Design review of the part built by this model. Coordinates are the model's own, in mm. A direction names the side the tool comes from. Coordinates: 2 decimals unless noted, no trailing zeros. Order: outer loops, then holes, each group sorted by start corner. A loop starts at its lowest first (then second) coordinate and runs counter-clockwise, first axis right, second up. Notation, with made-up numbers: (88.25, 33) - (121.25, 33) arc R12 ccw to (121.25, 52) - close; hole circle Ø4 at (22, -10.5). An arc over 180 degrees is marked (long way). Write item = value, one per line. Start each with the question number.
```python
from build123d import *

# Parameters (mm, degrees)
SKETCH_1_R               = 8.5
EXTRUDE_1_DEPTH          = 15
SKETCH_2_R               = 10
EXTRUDE_2_DEPTH          = 10
SKETCH_3_R               = 1
CUT_EXTRUDE_1_DEPTH      = 10
CUT_EXTRUDE_START        = -1.9
SKETCH_4_R               = 8.5
SKETCH_4_R_2             = 8.1
CUT_EXTRUDE_2_DEPTH      = 1.6
CHAMFER_1_SIZE           = 0.5
SKETCH_7_R               = 1
CUT_EXTRUDE_3_DEPTH      = 8
PATTERN_CIRCULAR_1_COUNT = 4
SKETCH_8_R               = 3.5
CUT_EXTRUDE_4_DEPTH      = 5.5
CHAMFER_2_SIZE           = 0.5
CUT_EXTRUDE_5_REACH      = 21.5
SKETCH_9_R               = 2.5


with BuildPart() as part:
    # Эскиз1 → Бобышка-Вытянуть1 (new body)
    with BuildSketch(Plane(origin=(0, 0, 0), x_dir=(1, 0, 0), z_dir=(0, 1, 0))):
        Circle(SKETCH_1_R)
    extrude(amount=EXTRUDE_1_DEPTH)

    # Эскиз2 → Бобышка-Вытянуть2 (add)
    with BuildSketch(Plane(origin=(0, 15, 0), x_dir=(1, 0, 0), z_dir=(0, 1, 0))):
        Circle(SKETCH_2_R)
    extrude(amount=EXTRUDE_2_DEPTH)

    # Эскиз3 → Вырез-Вытянуть1 (cut)
    with BuildSketch(Plane.XZ):
        with Locations((0, 6)):
            Circle(SKETCH_3_R)
        with Locations((6, 0)):
            Circle(SKETCH_3_R)
        with Locations((0, -6)):
            Circle(SKETCH_3_R)
        with Locations((-6, 0)):
            Circle(SKETCH_3_R)
    extrude(amount=-CUT_EXTRUDE_1_DEPTH, mode=Mode.SUBTRACT)

    # Эскиз4 → Вырез-Вытянуть2 (cut)
    with BuildSketch(Plane.XZ.offset(CUT_EXTRUDE_START)):
        Circle(SKETCH_4_R)
        Circle(SKETCH_4_R_2, mode=Mode.SUBTRACT)
    extrude(amount=-CUT_EXTRUDE_2_DEPTH, mode=Mode.SUBTRACT)

    # Фаска1
    chamfer_1_edges = [part.edges().sort_by_distance(p)[0] for p in [
        (-8.5, 0, 0),
        (-10, 25, 0),
    ]]
    chamfer(chamfer_1_edges, length=CHAMFER_1_SIZE)

    # Эскиз7 → Вырез-Вытянуть3 (cut)
    with BuildSketch(Plane(origin=(6.524591557, 0, 7.578238913), x_dir=(0.757823891, 0, -0.652459156), z_dir=(0.652459156, 0, 0.757823891))):
        with Locations((0, 22)):
            Circle(SKETCH_7_R)
    cut_extrude_3 = extrude(amount=-CUT_EXTRUDE_3_DEPTH, mode=Mode.SUBTRACT)

    # Круговой массив1: Вырез-Вытянуть3 ×4 about axis
    pattern_circular_1_axis = Axis((0, 0, 0), (0, 1, 0))
    for i in range(1, PATTERN_CIRCULAR_1_COUNT):
        add(cut_extrude_3.rotate(pattern_circular_1_axis, i * 360 / PATTERN_CIRCULAR_1_COUNT), mode=Mode.SUBTRACT)

    # Эскиз8 → Вырез-Вытянуть4 (cut)
    with BuildSketch(Plane.XZ):
        Circle(SKETCH_8_R)
    extrude(amount=-CUT_EXTRUDE_4_DEPTH, mode=Mode.SUBTRACT)

    # Фаска2
    chamfer_2_edges = [part.edges().sort_by_distance(p)[0] for p in [
        (-3.5, 0, 0),
    ]]
    chamfer(chamfer_2_edges, length=CHAMFER_2_SIZE)

    # Эскиз9 → Вырез-Вытянуть5 (cut, up to next)
    with BuildSketch(Plane.XZ.offset(-5.5), mode=Mode.PRIVATE) as cut_extrude_5_sk1:
        Circle(SKETCH_9_R)
    cut_extrude_5_tool1 = extrude(cut_extrude_5_sk1.sketch, amount=-CUT_EXTRUDE_5_REACH, mode=Mode.PRIVATE) & part.part
    add(cut_extrude_5_tool1.solids().sort_by_distance((0, 5.5, 0))[0], mode=Mode.SUBTRACT)


solid = part.part
```
Item 1: Add section C-C on y = 10.5. Give the boundary of the cut face in (x, z).
Item 2: For line 1 (Z direction, x = 0, y = 5); line 2 (Z direction, x = 0, y = 17); line 3 (X direction, y = 7.75, z = 0.5), list the stretches that pass through material, from the lowest coordinate up.
Item 3: For faces 4 (the cylindrical face through (-1.756, 2.689, -7.907)), 5 (the cylindrical face through (9.54, 19.68, -3)), 6 (the flat face through (0, 10, -6)), list the 3-axis set-ups (+Z, -Z, +X, -X, +Y, -Y) from which the entire face can be reached by the end or side of a thin tool; tool diameter is ignored.
Item 4: Mouldability with a two-part tool opening along Z and no side actions: class faces 1 (the flat face through (2, 0, -4)), 2 (the cylindrical face through (4.57, 9.17, -7.167)), 3 (the cylindrical face through (-0.54, 15.11, -2.44)) as +Z half, -Z half, draft (parallel to the pull), parting line (faces both ways), or undercut.
Item 5: Add section A-A on y = 3. Give the boundary of the cut face in (x, z), plus the area to 3 significant figures.
Item 6: Add section B-B on y = 17.25. Give the boundary of the cut face in (x, z), plus the area to 3 significant figures.
Item 7: For P1, Ø0.6, axis at x = -6, z = -0.5, coming from the -Y side; P2, Ø5, axis at x = -7, y = 3.5, coming from the -Z side; P3, Ø1.5, axis at x = 5, y = 10.5, coming from the +Z side, all flat-tipped, find the tip position at first contact; note any pin that passes through.
Worked out:
q1.outline = circle Ø17 at (0, 0); hole circle Ø5 at (0, 0)
q2.line_1 = -8.5 to -7, -5 to -3.5, 3.5 to 5, 7 to 8.5
q2.line_2 = -10 to -2.5, 2.5 to 10
q2.line_3 = -8.49 to -6.87, -5.13 to -2.45, 2.45 to 5.13, 6.87 to 8.49
q3.face_4 = none
q3.face_5 = +Y, -Y
q3.face_6 = -Y
q4.face_1 = draft
q4.face_2 = parting line
q4.face_3 = undercut
q5.outline = circle Ø16.2 at (0, 0); hole circle Ø2 at (-6, 0); hole circle Ø7 at (0, 0); hole circle Ø2 at (0, -6); hole circle Ø2 at (0, 6); hole circle Ø2 at (6, 0)
q5.area = 155 mm2
q6.outline = circle Ø20 at (0, 0); hole circle Ø5 at (0, 0)
q6.area = 295 mm2
q7.P1 = 10
q7.P2 = -7.21
q7.P3 = 7.36
